```python
from build123d import *

# Parameters (mm, degrees)
BOSS_EXTRUDE5_DEPTH = 5
BOSS_EXTRUDE6_DEPTH = 30
SKETCH4_R           = 4
SKETCH4_R_2         = 5
CUT_EXTRUDE1_DEPTH  = 30
SKETCH5_R           = 2.5
CUT_EXTRUDE2_DEPTH  = 30
SKETCH6_R           = 2.5
BOSS_EXTRUDE8_DEPTH = 30


with BuildPart() as part:
    # Sketch1 → Boss-Extrude5 (new body)
    with BuildSketch(Plane(origin=(0, 0, 0), x_dir=(1, 0, 0), z_dir=(0, 1, 0))):
        with BuildLine():
            Line((-43.995148291, 21.997574146), (-43.995148291, 0))
            Line((-43.995148291, 0), (-43.995148291, -21.997574146))
            Line((-43.995148291, -21.997574146), (-33.402902563, -21.997574146))
            ThreePointArc((-33.402902563, -21.997574146), (39.989521092, 0), (-33.402902563, 21.997574146))
            Line((-33.402902563, 21.997574146), (-43.995148291, 21.997574146))
        make_face()
    extrude(amount=BOSS_EXTRUDE5_DEPTH)

    # Sketch3 → Boss-Extrude6 (add)
    with BuildSketch(Plane(origin=(0, 5, 0), x_dir=(1, 0, 0), z_dir=(0, 1, 0))):
        with BuildLine():
            Line((-43.995148291, -21.997574146), (-33.402902563, -21.997574146))
            ThreePointArc((-33.402902563, -21.997574146), (39.989521092, 0), (-33.402902563, 21.997574146))
            Line((-33.402902563, 21.997574146), (-43.995148291, 21.997574146))
            Line((-43.995148291, 21.997574146), (-43.995148291, -21.997574146))
        make_face()
        with BuildLine():
            Line((-41, 19.004191941), (-31.749015624, 19.004191941))
            ThreePointArc((-31.749015624, 19.004191941), (36.998253479, 0.000315282), (-31.75, -19))
            Line((-31.75, -19), (-41, -19))
            Line((-41, -19), (-41, 19.004191941))
        make_face(mode=Mode.SUBTRACT)
    extrude(amount=BOSS_EXTRUDE6_DEPTH)

    # Sketch4 → Cut-Extrude1 (cut)
    with BuildSketch(Plane(origin=(0, 5, 0), x_dir=(1, 0, 0), z_dir=(0, 1, 0))):
        with Locations(Location((-22, 0, 0), (0, 0, 270))):
            Circle(SKETCH4_R)
        with Locations(Location((-21, 21, 0), (0, 0, 270))):
            Circle(SKETCH4_R_2)
        with Locations(Location((21, 21, 0), (0, 0, 270))):
            Circle(SKETCH4_R_2)
        with Locations(Location((21, -21, 0), (0, 0, 270))):
            Circle(SKETCH4_R_2)
        with Locations(Location((-21, -21, 0), (0, 0, 270))):
            Circle(SKETCH4_R_2)
    extrude(amount=-CUT_EXTRUDE1_DEPTH, mode=Mode.SUBTRACT)

    # Sketch5 → Cut-Extrude2 (cut)
    with BuildSketch(Plane(origin=(0, 5, 0), x_dir=(1, 0, 0), z_dir=(0, 1, 0))):
        with Locations(Location((-11, 32.25, 0), (0, 0, 270))):
            Circle(SKETCH5_R)
        with Locations(Location((11, 32.25, 0), (0, 0, 270))):
            Circle(SKETCH5_R)
        with Locations(Location((32.25, -11, 0), (0, 0, 270))):
            Circle(SKETCH5_R)
        with Locations(Location((32.25, 11, 0), (0, 0, 270))):
            Circle(SKETCH5_R)
        with Locations(Location((11, -32.25, 0), (0, 0, 270))):
            Circle(SKETCH5_R)
        with Locations(Location((-11, -32.25, 0), (0, 0, 270))):
            Circle(SKETCH5_R)
    extrude(amount=-CUT_EXTRUDE2_DEPTH, mode=Mode.SUBTRACT)

    # Sketch6 → Boss-Extrude8 (add)
    # profile 1 of 6: a face of its own
    with BuildSketch(Plane(origin=(0, 5, 0), x_dir=(1, 0, 0), z_dir=(0, 1, 0))):
        with BuildLine():
            ThreePointArc((-13.818927057, 34.324524101), (-12.091731491, 28.92462448), (-7.5, 32.25))
            ThreePointArc((-7.5, 32.25), (-8.205027171, 34.356686233), (-10.036072506, 35.614646161))
            ThreePointArc((-10.036072506, 35.614646161), (-11.944932636, 35.020701186), (-13.818927057, 34.324524101))
        make_face()
        with Locations(Location((-11, 32.25, 0), (0, 0, 270))):
            Circle(SKETCH6_R, mode=Mode.SUBTRACT)
    # profile 2 of 6: a face of its own
    with BuildSketch(Plane(origin=(0, 5, 0), x_dir=(1, 0, 0), z_dir=(0, 1, 0))):
        with BuildLine():
            ThreePointArc((13.820396396, 34.322526036), (11.94483736, 35.019542221), (10.034341301, 35.614149711))
            ThreePointArc((10.034341301, 35.614149711), (8.894032936, 29.454485249), (14.5, 32.25))
            ThreePointArc((14.5, 32.25), (14.325762122, 33.340553212), (13.820396396, 34.322526036))
        make_face()
        with Locations(Location((11, 32.25, 0), (0, 0, 270))):
            Circle(SKETCH6_R, mode=Mode.SUBTRACT)
    # profile 3 of 6: a face of its own
    with BuildSketch(Plane(origin=(0, 5, 0), x_dir=(1, 0, 0), z_dir=(0, 1, 0))):
        with BuildLine():
            ThreePointArc((35.613053698, 10.030531162), (35.017865848, 11.943917844), (34.319964959, 13.822276575))
            ThreePointArc((34.319964959, 13.822276575), (28.937333966, 9.870290414), (35.613053698, 10.030531162))
        make_face()
        with Locations(Location((32.25, 11, 0), (0, 0, 270))):
            Circle(SKETCH6_R, mode=Mode.SUBTRACT)
    # profile 4 of 6: a face of its own
    with BuildSketch(Plane(origin=(0, 5, 0), x_dir=(1, 0, 0), z_dir=(0, 1, 0))):
        with BuildLine():
            ThreePointArc((34.318509264, -13.82334366), (35.017020802, -11.943848204), (35.612690699, -10.029272818))
            ThreePointArc((35.612690699, -10.029272818), (28.937413903, -9.870056041), (34.318509264, -13.82334366))
        make_face()
        with Locations(Location((32.25, -11, 0), (0, 0, 270))):
            Circle(SKETCH6_R, mode=Mode.SUBTRACT)
    # profile 5 of 6: a face of its own
    with BuildSketch(Plane(origin=(0, 5, 0), x_dir=(1, 0, 0), z_dir=(0, 1, 0))):
        with BuildLine():
            ThreePointArc((10.02986849, -35.612862598), (11.943992144, -35.017283262), (13.82305009, -34.318909904))
            ThreePointArc((13.82305009, -34.318909904), (14.326460229, -33.338421951), (14.5, -32.25))
            ThreePointArc((14.5, -32.25), (8.895892147, -29.453085603), (10.02986849, -35.612862598))
        make_face()
        with Locations(Location((11, -32.25, 0), (0, 0, 270))):
            Circle(SKETCH6_R, mode=Mode.SUBTRACT)
    # profile 6 of 6: a face of its own
    with BuildSketch(Plane(origin=(0, 5, 0), x_dir=(1, 0, 0), z_dir=(0, 1, 0))):
        with BuildLine():
            ThreePointArc((-13.821585883, -34.320906348), (-11.944087605, -35.018442073), (-10.031594901, -35.61336016))
            ThreePointArc((-10.031594901, -35.61336016), (-8.203625754, -34.354825664), (-7.5, -32.25))
            ThreePointArc((-7.5, -32.25), (-12.089598414, -28.923924941), (-13.821585883, -34.320906348))
        make_face()
        with Locations(Location((-11, -32.25, 0), (0, 0, 270))):
            Circle(SKETCH6_R, mode=Mode.SUBTRACT)
    extrude(amount=BOSS_EXTRUDE8_DEPTH)


solid = part.part
```
Geometry check sheet. Reference: the model listing, model coordinates, mm. A direction names the side the tool comes from. Coordinates: 2 decimals unless noted, no trailing zeros. Order: outer loops, then holes, each group sorted by start corner. A loop starts at its lowest first (then second) coordinate and runs counter-clockwise, first axis right, second up. Notation, with made-up numbers: (4.25, -30.75) - (32.25, -30.75) arc R20 ccw to (32.25, 7.25) - close; hole circle Ø8 at (2, -37). An arc over 180 degrees is marked (long way). Answer in a Markdown table with one row per item. Add a question column.
1. Section check A-A (y = 12). Enter the section's corners in (x, z), plus the area to 3 significant figures.
2. Access from +Z, -Z, +X, -X, +Y, -Y to the whole of each face (thin tool, end or side, straight path). Record for faces 1 (the face through (-36, 20, 19)), 2 (the face through (-39, 17, -21.998)), 3 (the face through (39.964, 17.255, 1.433)).
3. Section check C-C (z = -21). Enter the section's corners in (x, y), plus the area to 3 significant figures.
4. Gauge pin test, flat ends, axial feed: pin 1 Ø1 at (y, z) = (4.5, 8.5) entering from +X; pin 2 Ø6 at (x, z) = (21, 21) entering from -Y; pin 3 Ø1.5 at (y, z) = (6, -5) entering from +X; pin 4 Ø3 at (y, z) = (28, -4.5) entering from +X. Record the tip position at first contact, or that the pin passes through.
5. Draft check along Z on faces 4 (the face through (-39, 17, 21.998)), 5 (the face through (-43.995, 17, 0)), 6 (the face through (-23.911, 19.79, 28.236)). Enter one of: +Z half, -Z half, draft (parallel to the pull), parting line (faces both ways), or undercut.
6. Section check B-B (x = -22). Enter the section's corners in (y, z), plus the area to 3 significant figures.
7. Section check D-D (x = 20). Enter the section's corners in (y, z).
8. Material ranges on L1, parallel to X at y = 3.5, z = 32; L2, parallel to X at y = 16.5, z = -32.25; L3, parallel to Z at x = 0, y = 24, recorded low to high. Write a range as [from, to].
Data:
| question | item | result |
|---|---|---|
| 1 | outline | (-44, -22) - (-33.4, -22) arc R39.99 ccw (long way) to (-33.4, 22) - (-44, 22) - close; hole (-41, -19) - (-31.75, -19) arc R37 ccw to (-13.82, -34.32) arc R3.5 cw (long way) to (-10.04, -35.61) arc R37 ccw to (10.03, -35.61) arc R3.5 cw (long way) to (13.82, -34.32) arc R37 ccw to (34.32, -13.82) arc R3.5 cw (long way) to (35.61, -10.03) arc R37 ccw to (35.61, 10.03) arc R3.5 cw (long way) to (34.32, 13.82) arc R37 ccw to (13.82, 34.32) arc R3.5 cw (long way) to (10.03, 35.61) arc R37 ccw to (-10.03, 35.61) arc R3.5 cw (long way) to (-13.82, 34.32) arc R37 ccw to (-31.75, 19) - (-41, 19) - close; hole circle Ø5 at (-11, -32.25); hole circle Ø5 at (-11, 32.25); hole circle Ø5 at (11, -32.25); hole circle Ø5 at (11, 32.25); hole circle Ø5 at (32.25, -11); hole circle Ø5 at (32.25, 11) |
| 1 | area | 880 mm² |
| 2 | face 1 | +Y |
| 2 | face 2 | -Z, -X, +Y, -Y |
| 2 | face 3 | +Y, -Y |
| 3 | outline | (-44, 0) - (-26, 0) - (-26, 5) - (-30.47, 5) - (-30.47, 35) - (-44, 35) - close; (-16, 0) - (16, 0) - (16, 5) - (-16, 5) - close; (26, 0) - (34.03, 0) - (34.03, 35) - (30.46, 35) - (30.46, 5) - (26, 5) - close |
| 3 | area | 803 mm² |
| 4 | pin 1 | stops at x = 39.18 |
| 4 | pin 2 | passes through |
| 4 | pin 3 | stops at x = 39.76 |
| 4 | pin 4 | stops at x = 39.88 |
| 5 | face 4 | +Z half |
| 5 | face 5 | draft |
| 5 | face 6 | undercut |
| 6 | outline | (0, -33.4) - (35, -33.4) - (35, -29.75) - (5, -29.75) - (5, -25.9) - (0, -25.9) - close; (0, -16.1) - (5, -16.1) - (5, -4) - (0, -4) - close; (0, 4) - (5, 4) - (5, 16.1) - (0, 16.1) - close; (0, 25.9) - (5, 25.9) - (5, 29.75) - (35, 29.75) - (35, 33.4) - (0, 33.4) - close |
| 6 | area | 415 mm² |
| 7 | outline | (0, -34.63) - (35, -34.63) - (35, -31.13) - (5, -31.13) - (5, -25.9) - (0, -25.9) - close; (0, -16.1) - (5, -16.1) - (5, 16.1) - (0, 16.1) - close; (0, 25.9) - (5, 25.9) - (5, 31.13) - (35, 31.13) - (35, 34.63) - (0, 34.63) - close |
| 8 | L1 | x = [-23.99, -13.49], [-8.51, 8.51], [13.49, 23.98] |
| 8 | L2 | x = [-23.65, -18.14], [-14.5, -13.5], [-8.5, -7.5], [7.5, 8.5], [13.5, 14.5], [18.14, 23.65] |
| 8 | L3 | z = [-39.99, -37], [37, 39.99] |
